Autodesk Inventor part; units mm, degrees
ref_plane "YZ Plane" through (0, 0, 0) normal (1, 0, 0) x (0, 1, 0)
ref_plane "XZ Plane" through (0, 0, 0) normal (0, 1, 0) x (-1, 0, 0)
ref_plane "XY Plane" through (0, 0, 0) normal (0, 0, 1) x (1, 0, 0)
sketch "Sketch1" plane through (0, 0, 0) normal (0, 1, 0) x (-1, 0, 0)
  line L0 (-0.9998, -14.9003) -> (-26.9998, -14.9003)
  line L1 (-26.9998, -14.9003) -> (-26.9998, -22.9003)
  line L2 (-26.9998, -22.9003) -> (-0.9998, -22.9003)
  line L3 (-0.9998, -22.9003) -> (-0.9998, -14.9003)
  line L4 (-0.9998, -14.9003) -> (-8.9998, -14.9003)
  line L5 (-8.9998, -14.9003) -> (-8.9998, -10.9694)
  line L6 (-8.9998, -10.9694) -> (-0.9998, -10.9694) construction
  line L7 (-0.9998, -10.9694) -> (-0.9998, -14.9003)
  line L8 (13.404, 6.5843) -> (26.404, -15.9324)
  line L9 (26.404, -15.9324) -> (33.3322, -11.9324)
  line L10 (33.3322, -11.9324) -> (20.3322, 10.5843)
  line L11 (20.3322, 10.5843) -> (13.404, 6.5843)
  line L12 (13.404, 6.5843) -> (17.404, -0.3439)
  line L13 (17.404, -0.3439) -> (13.9997, -2.3094)
  line L14 (13.9997, -2.3094) -> (9.9997, 4.6188) construction
  line L15 (9.9997, 4.6188) -> (13.404, 6.5843)
  line L16 (-12.4041, 8.316) -> (0.5959, 30.8327)
  line L17 (0.5959, 30.8327) -> (-6.3323, 34.8327)
  line L18 (-6.3323, 34.8327) -> (-19.3323, 12.316)
  line L19 (-19.3323, 12.316) -> (-12.4041, 8.316)
  line L20 (-12.4041, 8.316) -> (-8.4041, 15.2442)
  line L21 (-8.4041, 15.2442) -> (-4.9998, 13.2788)
  line L22 (-4.9998, 13.2788) -> (-8.9998, 6.3506) construction
  line L23 (-8.9998, 6.3506) -> (-12.4041, 8.316)
  line L24 (17.9997, 0) -> (-8.9998, -15.5882)
  line L25 (-8.9998, -15.5882) -> (-8.9998, 15.5882)
  line L26 (-8.9998, 15.5882) -> (17.9997, 0)
  point P0 (0, 0)
  point P1 (0, 0)
  point P2 (17.404, -0.3439)
  dimension "d0" = 8
  dimension "d3" = 360
  dimension "d5" = 60.332
  dimension "d6" = 57.733
  dimension "d7" = 26
extrude "Extrusion1" add sketch "Sketch1" along normal blind 8
fillet "Fillet1" radius 4 3 edges at (8.9998, 4, 6.3506) (-9.9997, 4, 4.6188) (0.9998, 4, -10.9694)
sketch "Sketch2" plane through (0, 8, 0) normal (0, 1, 0) x (1, 0, 0)
  line L0 (8.9998, -4.0412) -> (8.9998, 14.9003)
  circle A0 centre (8.9998, 14.9003) radius 2
  line L1 (8.4041, -15.2442) -> (-0.5959, -30.8327)
  circle A1 centre (8.4041, -15.2442) radius 2
  line L2 (-1.0002, 9.8147) -> (-17.404, 0.3439)
  circle A2 centre (-17.404, 0.3439) radius 2
  circle A3 centre (0, 0) radius 4.25
  dimension "d11" = 4
  dimension "d14" = 8.5
extrude "Extrusion2" cut sketch "Sketch2" against normal blind 18.75
chamfer "Chamfer1" distance 4.5 angle 45 1 edges at (-4.25, 8, 0)
sketch "Sketch3" plane through (26.9998, 0, -22.9003) normal (0, 0, -1) x (-1, 0, 0)
  circle A0 centre (4, 4) radius 2.5
  circle A1 centre (14, 4) radius 2.5
  line L0 (0, 0) -> (26, 0)
  line L1 (0, 0) -> (0, 8)
  point P0 (26.9998, 0)
  dimension "d18" = 10
  dimension "d19" = 5
  dimension "d20" = 4
  dimension "d21" = 4
extrude "Extrusion3" cut sketch "Sketch3" against normal blind 18.75
thread "Thread1"
thread "Thread2"
pattern_circular "Circular Pattern1" count 3 over 360 about axis through (0, 8, 0) along (0, -1, 0) of "Extrusion3"
thread "Thread3"
thread "Thread4"
thread "Thread5"
thread "Thread6"
properties part number "ServoCap" material "Steel, Carbon"
Build history of the part. All positions in model axes, mm. A direction names the side the tool comes from. Give positions to 0.01 mm unless a question says otherwise; leave off trailing zeros. Loops run counter-clockwise (first coordinate to the right, second up) from the corner with the lowest first, then second, coordinate; pieces in that order, holes last. Notation, with made-up numbers: (69, -18) - (108, -18) arc R13 ccw to (108, 0) - close; hole circle Ø10 at (39.5, 22.25). An arc over 180 degrees is marked (long way). Write item = value, one per line. Start each with the question number.
1) Band-saw the part on C-C on z = 15.5. Give the cut face in (x, y).
2) Probe probe 1 along Z at (x, y) = (9.5, 3.5); probe 2 along Z at (x, y) = (-0.5, 0.75); probe 3 along X at (y, z) = (3.25, -1). List the from-to ranges inside material, lowest first. Write a range as from..to.
3) Band-saw the part on D-D on x = -10. Give the cut face in (y, z), plus the area to 4 significant figures.
4) Drop flat-ended pins along their axis: pin 1 Ø1 at (y, z) = (2, -11.5) entering from +X; pin 2 Ø2.5 at (x, y) = (23, 2.5) entering from +Z; pin 3 Ø2 at (x, y) = (-1.5, 4) entering from -Z. Give the stop position or say it passes through.
5) Tool access for faces 1 (the cylindrical face through (9.521, 4.056, 6.016)), 2 (the flat face through (3.46, 3.94, 23.81)), 3 (the flat face through (-22.35, 3.94, -8.91)), 4 (the cylindrical face through (-24.17, 4.11, -3.94)): list every direction of +Z, -Z, +X, -X, +Y, -Y with a clear straight run to the whole face (end or side of a thin tool).
6) Pull direction Z, two halves, no side cores. Call faces 5 (the flat face through (27, 4, -19)), 6 (the flat face through (2.82, 3.944, 32.805)), 7 (the cylindrical face through (10.35, 4.06, 14.79)): +Z half, -Z half, draft (parallel to the pull), parting line (faces both ways), or undercut.
7) Band-saw the part on A-A on x = 18.5. Give the cut face in (y, z), plus the area to 3 significant figures.
8) Band-saw the part on B-B on z = 0. Count the separate pieces of the cut face and the enclosed holes in it, plus the area to 3 significant figures.
Final values:
q1.outline = (10.39, 0) - (17.49, 0) - (17.49, 8) - (10.39, 8) - close
q2.probe_1 = -22.9..-16.84, 5.98..13.57, 16.92..17.67, 23.32..29.21
q2.probe_2 = -10.16..-4.22, 4.22..10.1, 30.67..30.89
q2.probe_3 = -19.5..-19.29, -15.51..-4.13, 4.13..9
q3.outline = (0, -4.62) - (8, -4.62) - (8, 5.24) - (0, 5.24) - close
q3.area = 78.85 mm²
q4.pin_1 = 9
q4.pin_2 = -14.9
q4.pin_3 = -10.16
q5.face_1 = +X, +Y, -Y
q5.face_2 = -X, +Y, -Y
q5.face_3 = -Z, +Y, -Y
q5.face_4 = none
q6.face_5 = draft
q6.face_6 = +Z half
q6.face_7 = undercut
q7.outline = (0, -22.9) - (8, -22.9) - (8, -14.9) - (0, -14.9) - close; (0, 11.84) - (8, 11.84) - (8, 13.76) - (0, 13.76) - close
q7.area = 79.4 mm²
q8.separate_pieces = 3
q8.enclosed_holes = 0
q8.area = 142 mm²
